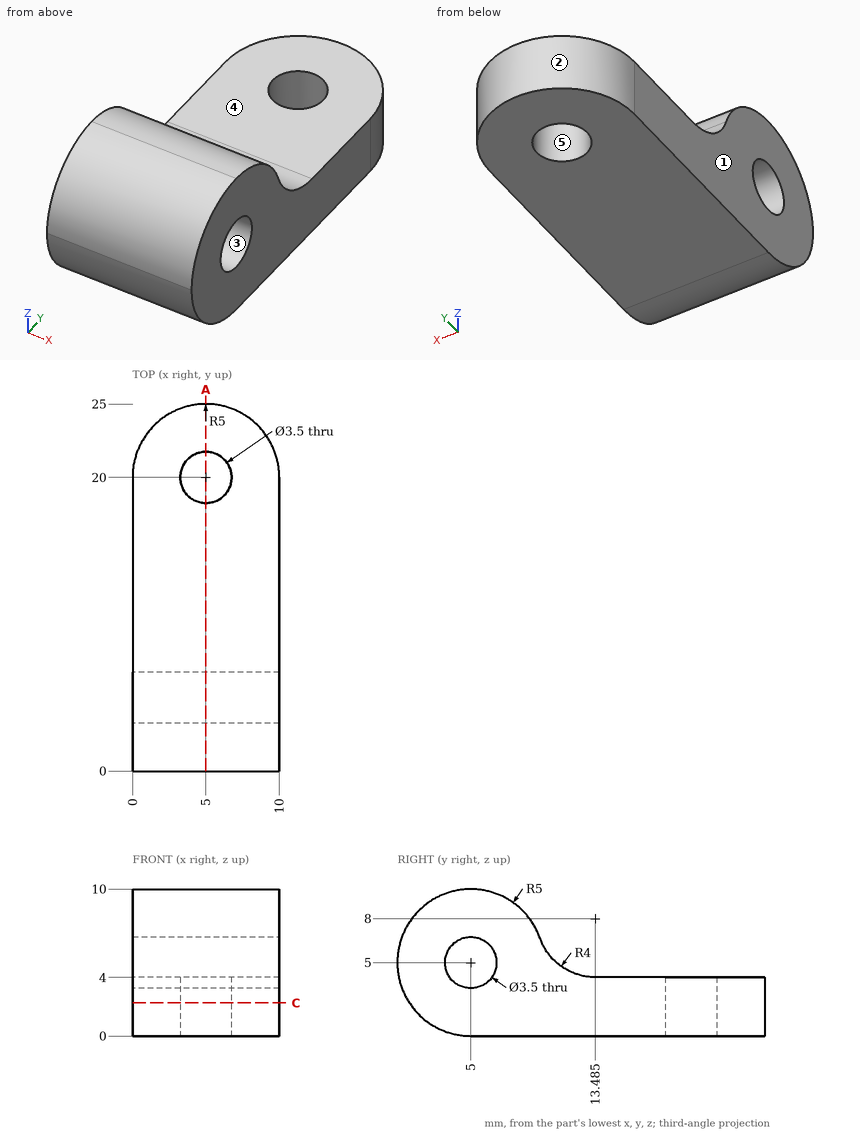
Source: three-view drawing plus pictorial views. Frame: mm from the lowest corner of the part. A direction names the side the tool comes from. Round coordinates to 2 decimals unless told otherwise and drop trailing zeros. Order: outer loops, then holes, each group sorted by start corner. A loop starts at its lowest first (then second) coordinate and runs counter-clockwise, first axis right, second up. Notation, with made-up numbers: (78.25, -32.75) -> (109.25, -32.75) arc R24 cw to (109.25, -20.75) -> close; hole circle Ø2 at (75, -25). An arc over 180 degrees is marked (long way). Use CSV: the item, a comma, the result in double quotes. Start each with the question number.
1) Draft query along Y for the marked faces 1, 2 and 3. Return one class per face: +Y half, -Y half, draft (parallel to the pull), parting line (faces both ways), or undercut.
2) Section C-C (z = 2.25). Return the cut outline in (x, y).
3) Material intervals for line 1 along X through (y, z) = (20, 2.4); line 2 along Z through (x, y) = (5.75, 16); line 3 along Y through (x, z) = (6.25, 6.5) (1 decimal), sorted ascending. Write a range as from..to.
4) Set-up query: the marked faces 4 and 5. Return all of +Z, -Z, +X, -X, +Y, -Y with unobstructed straight access to the full face (end or side cutting, diameter ignored); none if empty.
5) Section A-A (x = 5). State how many separate pieces and enclosed holes the cut face has, and give its area (3 significant figures).
6) First-contact query: pin 1 Ø1 at (x, y) = (7, 18.5) entering from +Z; pin 2 Ø1.5 at (x, z) = (5.5, 7.5) entering from -Y; pin 3 Ø3 at (x, y) = (1.5, 8) entering from +Z. Flat tips, straight axial feed; report the tip coordinate or a pass-through.
Returned:
1,face 1,"draft"
1,face 2,"+Y half"
1,face 3,"undercut"
2,outline,"(0, 0.82) -> (10, 0.82) -> (10, 20) arc R5 ccw to (0, 20) -> close; hole circle Ø3.5 at (5, 20)"
3,line 1,"x = 0..3.25, 6.75..10"
3,line 2,"z = 0..4"
3,line 3,"y = 0.2..4.1, 5.9..9.8"
4,face 4,"+Z, +X, -X, +Y"
4,face 5,"+Z, -Z"
5,separate pieces,"2"
5,enclosed holes,"1"
5,area,"122 mm²"
6,pin 1,"stops at z = 4"
6,pin 2,"stops at y = 0.32"
6,pin 3,"stops at z = 9.77"
